Model file for the job. Use its own axes, mm. Face numbers are marked on the shaded views. A direction names the side the tool comes from. Give positions to 0.01 mm unless a question says otherwise; leave off trailing zeros. Order: outer loops, then holes, each group sorted by start corner. A loop starts at its lowest first (then second) coordinate and runs counter-clockwise, first axis right, second up. Notation, with made-up numbers: (13, 3) - (44, 3) arc R6 cw to (44, 7) - close; hole circle Ø7 at (-21.75, 59). An arc over 180 degrees is marked (long way). Return JSON: item names as keys, results as strings. Group by question number.
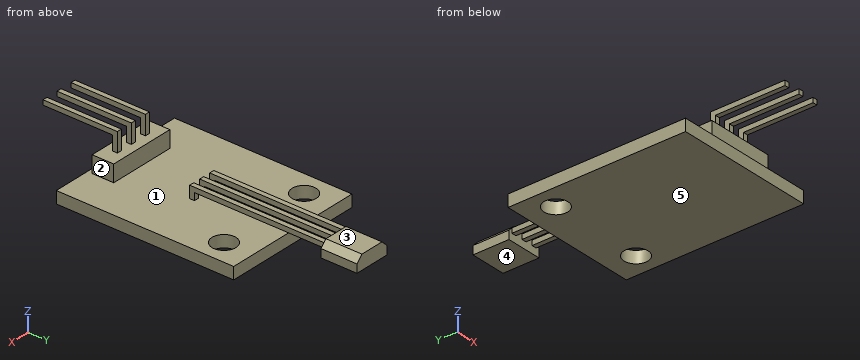
from build123d import *

# Parameters (mm, degrees)
SKETCH1_W               = 14.986
SKETCH1_H               = 18.796
BOSS_EXTRUDE1_DEPTH     = 0.635
SKETCH2_W               = 7.112
SKETCH2_H               = 2.286
BOSS_EXTRUDE2_DEPTH     = 1.778
SKETCH3_W               = 0.508
SKETCH3_H               = 0.508
BOSS_EXTRUDE3_DEPTH     = 2.032
SKETCH4_W               = 0.508
SKETCH4_H               = 0.508
BOSS_EXTRUDE4_DEPTH     = 7.366
CUT_EXTRUDE1_DEPTH      = 18.515873886
CUT_EXTRUDE1_DEPTH_BACK = 18.515873886
SKETCH5_R               = 1.27
SKETCH6_W               = 0.508
SKETCH6_H               = 0.508
BOSS_EXTRUDE5_DEPTH     = 1.27
SKETCH7_W               = 0.508
SKETCH7_H               = 0.508
BOSS_EXTRUDE6_DEPTH     = 13.716
LPATTERN1_COUNT         = 2
LPATTERN1_PITCH         = 1.27
MIRROR1_COPY_1_SKETCH_W = 0.508
MIRROR1_COPY_1_SKETCH_H = 0.508
MIRROR1_COPY_1_DEPTH    = 1.27
MIRROR1_COPY_2_SKETCH_W = 0.508
MIRROR1_COPY_2_SKETCH_H = 0.508
MIRROR1_COPY_2_DEPTH    = 13.716
MIRROR1_COPY_3_SKETCH_W = 0.508
MIRROR1_COPY_3_SKETCH_H = 0.508
MIRROR1_COPY_3_DEPTH    = 1.27
MIRROR1_COPY_4_SKETCH_W = 0.508
MIRROR1_COPY_4_SKETCH_H = 0.508
MIRROR1_COPY_4_DEPTH    = 13.716
SKETCH8_W               = 3.81
SKETCH8_H               = 1.524
BOSS_EXTRUDE7_DEPTH     = 3.81
CHAMFER1_SIZE           = 0.635


with BuildPart() as part:
    # Sketch1 → Boss-Extrude1 (new, symmetric)
    with BuildSketch(Plane.XY):
        Rectangle(SKETCH1_W, SKETCH1_H)
    extrude(amount=BOSS_EXTRUDE1_DEPTH, both=True)

    # Sketch2 → Boss-Extrude2 (add)
    with BuildSketch(Plane.XY.offset(0.635)):
        with Locations((0, -7.747)):
            Rectangle(SKETCH2_W, SKETCH2_H)
    extrude(amount=BOSS_EXTRUDE2_DEPTH)

    # Sketch3 → Boss-Extrude3 (add)
    with BuildSketch(Plane.XY.offset(2.413)):
        with Locations((-1.778, -7.747)):
            Rectangle(SKETCH3_W, SKETCH3_H)
        with Locations((0, -7.747)):
            Rectangle(SKETCH3_W, SKETCH3_H)
        with Locations((1.778, -7.747)):
            Rectangle(SKETCH3_W, SKETCH3_H)
    extrude(amount=BOSS_EXTRUDE3_DEPTH)

    # Sketch4 → Boss-Extrude4 (add)
    with BuildSketch(Plane.XZ.offset(8.001)):
        with Locations((-1.778, 4.191)):
            Rectangle(SKETCH4_W, SKETCH4_H)
        with Locations((0, 4.191)):
            Rectangle(SKETCH4_W, SKETCH4_H)
        with Locations((1.778, 4.191)):
            Rectangle(SKETCH4_W, SKETCH4_H)
    extrude(amount=BOSS_EXTRUDE4_DEPTH)

    # Sketch5 → Cut-Extrude1 (cut, two sides: drawn at the far end of the back side and taken through both)
    with BuildSketch(Plane.XY.offset(0.635).offset(-CUT_EXTRUDE1_DEPTH_BACK)):
        with Locations((-5.08, 6.35)):
            Circle(SKETCH5_R)
        with Locations((5.08, 6.35)):
            Circle(SKETCH5_R)
    extrude(amount=CUT_EXTRUDE1_DEPTH + CUT_EXTRUDE1_DEPTH_BACK, mode=Mode.SUBTRACT)

    # Sketch6 → Boss-Extrude5 (add)
    with BuildSketch(Plane.XY.offset(0.635)):
        Rectangle(SKETCH6_W, SKETCH6_H)
    boss_extrude5 = extrude(amount=BOSS_EXTRUDE5_DEPTH)

    # Sketch7 → Boss-Extrude6 (add)
    with BuildSketch(Plane(origin=(0, 0.254, 0), x_dir=(1, 0, 0), z_dir=(0, 1, 0))):
        with Locations((0, -1.651)):
            Rectangle(SKETCH7_W, SKETCH7_H)
    boss_extrude6 = extrude(amount=BOSS_EXTRUDE6_DEPTH)

    # LPattern1: Boss-Extrude5, Boss-Extrude6 ×2
    with Locations(*[(i * LPATTERN1_PITCH, 0, 0) for i in range(1, LPATTERN1_COUNT)]):
        add(boss_extrude5)
        add(boss_extrude6)

    # Mirror1 copy 1 sketch → Mirror1 copy 1 (add)
    with BuildSketch(Plane(origin=(-1.27, 0, 0.635), x_dir=(-1, 0, 0), z_dir=(0, 0, 1))):
        Rectangle(MIRROR1_COPY_1_SKETCH_W, MIRROR1_COPY_1_SKETCH_H)
    extrude(amount=MIRROR1_COPY_1_DEPTH)

    # Mirror1 copy 2 sketch → Mirror1 copy 2 (add)
    with BuildSketch(Plane(origin=(-1.27, 0.254, 0), x_dir=(-1, 0, 0), z_dir=(0, 1, 0))):
        with Locations((0, 1.651)):
            Rectangle(MIRROR1_COPY_2_SKETCH_W, MIRROR1_COPY_2_SKETCH_H)
    extrude(amount=MIRROR1_COPY_2_DEPTH)

    # Mirror1 copy 3 sketch → Mirror1 copy 3 (add)
    with BuildSketch(Plane(origin=(0, 0, 0.635), x_dir=(-1, 0, 0), z_dir=(0, 0, 1))):
        Rectangle(MIRROR1_COPY_3_SKETCH_W, MIRROR1_COPY_3_SKETCH_H)
    extrude(amount=MIRROR1_COPY_3_DEPTH)

    # Mirror1 copy 4 sketch → Mirror1 copy 4 (add)
    with BuildSketch(Plane(origin=(0, 0.254, 0), x_dir=(-1, 0, 0), z_dir=(0, 1, 0))):
        with Locations((0, 1.651)):
            Rectangle(MIRROR1_COPY_4_SKETCH_W, MIRROR1_COPY_4_SKETCH_H)
    extrude(amount=MIRROR1_COPY_4_DEPTH)

    # Sketch8 → Boss-Extrude7 (add)
    with BuildSketch(Plane(origin=(0, 13.97, 0), x_dir=(1, 0, 0), z_dir=(0, 1, 0))):
        with Locations((0, -1.397)):
            Rectangle(SKETCH8_W, SKETCH8_H)
    extrude(amount=BOSS_EXTRUDE7_DEPTH)

    # Chamfer1
    chamfer1_edges = [part.edges().sort_by_distance(p)[0] for p in [
        (1.905, 15.875, 2.159),
        (-1.905, 15.875, 2.159),
    ]]
    chamfer(chamfer1_edges, length=CHAMFER1_SIZE - 0.0001)  # a hair under: the kernel refuses the full size


solid = part.part
(1) Slice it at D-D (x = 2.75). Give the cut face in (y, z) (3 decimals).
(2) 3-axis set-ups, long thin cutter, end or side, ignore diameter. For the marked faces 3, 4 and 5: which of +Z, -Z, +X, -X, +Y, -Y reach the whole face in a straight line?
(3) Slice it at B-B (x = 5.08). Give the cut face in (y, z) (3 decimals), and give its area (3 significant figures).
(4) Pull direction Y, two halves, no side cores. Call the marked faces 1 and 2: released by +Y, released by -Y, zero draft, split by the parting line, or undercut.
(5) Slice it at C-C (y = 10). Give the cut face in (x, z) (3 decimals), and give its area (3 significant figures).
(6) Drill centre lines: L1, parallel to X at y = 6.35, z = -0.25; L2, parallel to Y at x = -5.08, z = -0.2; L3, parallel to Y at x = 0.5, z = 1.2. Where is each one in solid material? Low to high.
(7) Slice it at A-A (y = 6.35). Give the cut face in (x, z) (3 decimals).
(8) Drop flat-ended pins along their axis: pin 1 Ø0.6 at (x, z) = (0, 3) entering from +Y; pin 2 Ø1 at (x, z) = (-3, 1.5) entering from +Y; pin 3 Ø5 at (x, y) = (5.5, 6.5) entering from +Z (3 decimals). Give the stop position or say it passes through.
Result set:
{
 "1": {"outline": "(-9.398, -0.635) - (9.398, -0.635) - (9.398, 0.635) - (-6.604, 0.635) - (-6.604, 2.413) - (-8.89, 2.413) - (-8.89, 0.635) - (-9.398, 0.635) - close"},
 "2": {"face 3": "+Z, +X, -X, +Y", "face 4": "-Z, +X, -X, +Y", "face 5": "-Z, +X, -X, +Y, -Y"},
 "3": {"outline": "(-9.398, -0.635) - (5.08, -0.635) - (5.08, 0.635) - (-9.398, 0.635) - close; (7.62, -0.635) - (9.398, -0.635) - (9.398, 0.635) - (7.62, 0.635) - close", "area": "20.6 mm²"},
 "4": {"face 1": "undercut", "face 2": "zero draft"},
 "5": {"outline": "(-1.524, 1.397) - (-1.016, 1.397) - (-1.016, 1.905) - (-1.524, 1.905) - close; (-0.254, 1.397) - (0.254, 1.397) - (0.254, 1.905) - (-0.254, 1.905) - close; (1.016, 1.397) - (1.524, 1.397) - (1.524, 1.905) - (1.016, 1.905) - close", "area": "0.774 mm²"},
 "6": {"L1": "x = -7.49 to -6.35, -3.81 to 3.81, 6.35 to 7.49", "L2": "y = -9.4 to 5.08, 7.62 to 9.4", "L3": "y = -8.89 to -6.6, 13.97 to 17.78"},
 "7": {"outline": "(-7.493, -0.635) - (-6.35, -0.635) - (-6.35, 0.635) - (-7.493, 0.635) - close; (-3.81, -0.635) - (3.81, -0.635) - (3.81, 0.635) - (-3.81, 0.635) - close; (-1.524, 1.397) - (-1.016, 1.397) - (-1.016, 1.905) - (-1.524, 1.905) - close; (-0.254, 1.397) - (0.254, 1.397) - (0.254, 1.905) - (-0.254, 1.905) - close; (1.016, 1.397) - (1.524, 1.397) - (1.524, 1.905) - (1.016, 1.905) - close; (6.35, -0.635) - (7.493, -0.635) - (7.493, 0.635) - (6.35, 0.635) - close"},
 "8": {"pin 1": "stops at y = -7.49", "pin 2": "stops at y = -6.6", "pin 3": "stops at z = 0.635"}
}
